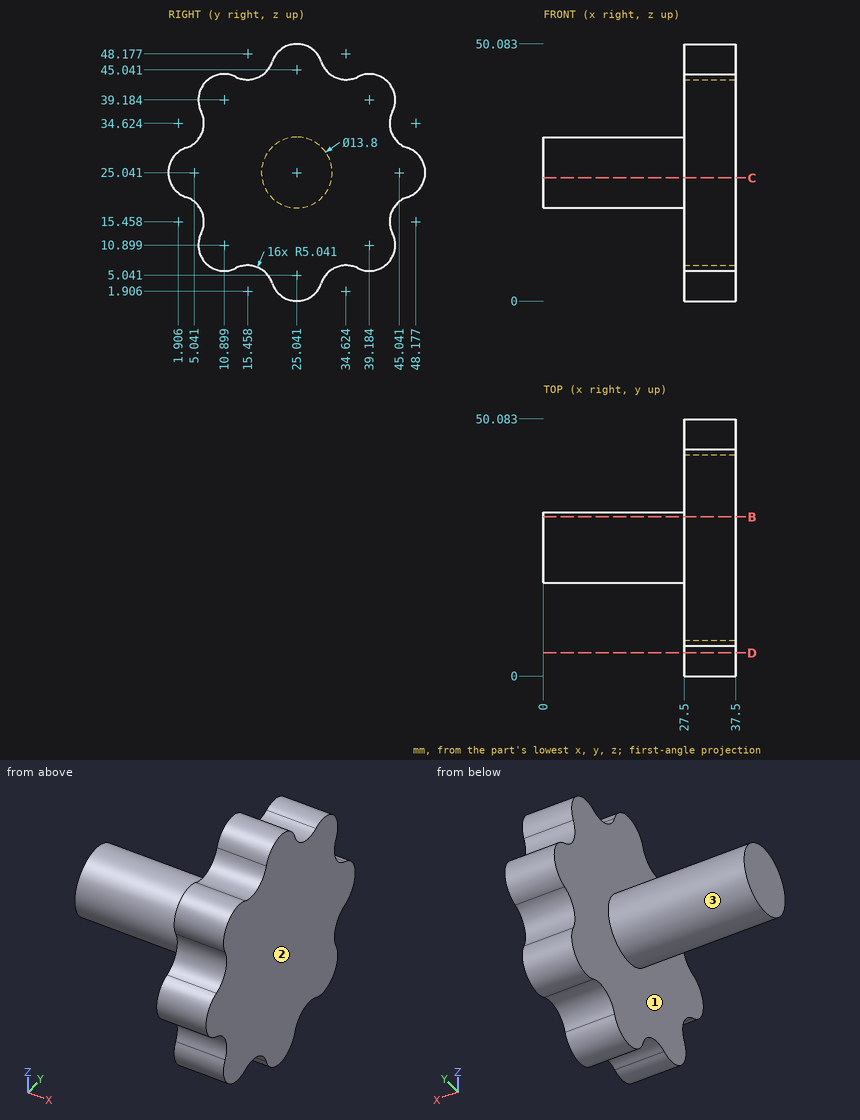
Study the drawing (mm; zero at the part's minimum x, y, z) and answer. Give positions to 0.01 mm unless a question says otherwise; leave off trailing zeros. Order: outer loops, then holes, each group sorted by start corner. A loop starts at its lowest first (then second) coordinate and runs counter-clockwise, first axis right, second up. Notation, with made-up numbers: (55.5, -29.5) - (84.5, -29.5) arc R23 cw to (84.5, -1.5) - close; hole circle Ø7 at (-36.5, -15). An arc over 180 degrees is marked (long way). Answer in a Markdown table with one row per item. Add a question column.
Q1. The part is cut by section B-B (y = 31). Determine the outline of the cut face in (x, z).
Q2. The part is cut by section C-C (z = 24). Determine the outline of the cut face in (x, y) (1 decimal).
Q3. Find the intervals of material crossed by line 1 along X through (y, z) = (30.5, 36); line 2 along Z through (x, y) = (16, 23); line 3 along Y through (x, z) = (32.5, 25.5), in increasing order. Write a range as [from, to].
Q4. For a pull along X with two mould halves and no side action, classify the marked faces 1, 2 and 3 as released by +X, released by -X, zero draft, split by the parting line, or undercut.
Q5. The part is cut by section D-D (y = 4.5). Determine the outline of the cut face in (x, z), then the cut area to 3 significant figures.
Q6. Given P1, Ø10, axis at y = 16.5, z = 20.5, coming from the -X side; P2, Ø2, axis at x = 23, y = 22.5, coming from the -Z side (1 decimal); P3, Ø8, axis at x = 4.5, y = 27.5, coming from the +Z side; P4, Ø1.5, axis at y = 38.5, z = 30.5, coming from the -X side, each flat-ended and moving along its own axis, determine where each tip first touches the part or whether it passes through.
Determined:
| question | item | result |
|---|---|---|
| 1 | outline | (0, 21.56) - (27.5, 21.56) - (27.5, 5.41) - (37.5, 5.41) - (37.5, 44.67) - (27.5, 44.67) - (27.5, 28.52) - (0, 28.52) - close |
| 2 | outline | (0, 18.2) - (27.5, 18.2) - (27.5, 0.1) - (37.5, 0.1) - (37.5, 50) - (27.5, 50) - (27.5, 31.9) - (0, 31.9) - close |
| 3 | line 1 | x = [27.5, 37.5] |
| 3 | line 2 | z = [18.45, 31.63] |
| 3 | line 3 | y = [0.02, 50.06] |
| 4 | face 1 | released by -X |
| 4 | face 2 | released by +X |
| 4 | face 3 | zero draft |
| 5 | outline | (27.5, 19.78) - (37.5, 19.78) - (37.5, 30.3) - (27.5, 30.3) - close |
| 5 | area | 105 mm² |
| 6 | P1 | stops at x = 0 |
| 6 | P2 | stops at z = 18.3 |
| 6 | P3 | stops at z = 31.94 |
| 6 | P4 | stops at x = 27.5 |
